Read the model definition and answer for the solid it produces. Units are mm, in the model's axes. Face numbers are marked on the shaded views. Give positions to 0.01 mm unless a question says otherwise; leave off trailing zeros. Order: outer loops, then holes, each group sorted by start corner. A loop starts at its lowest first (then second) coordinate and runs counter-clockwise, first axis right, second up.
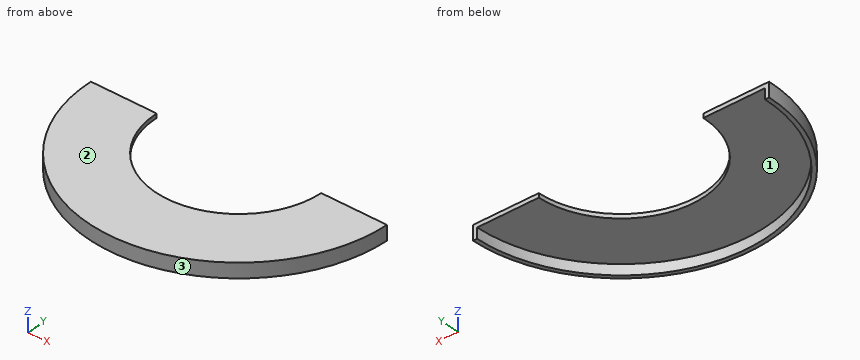
```python
from build123d import *

# Parameters (mm, degrees)
BOSS_EXTRUDE1_DEPTH = 5
BOSS_EXTRUDE2_DEPTH = 2


with BuildPart() as part:
    # Sketch1 → Boss-Extrude1 (new body)
    with BuildSketch(Plane.XY):
        with BuildLine():
            Line((72, 0), (70, 0))
            ThreePointArc((70, 0), (0, -70), (-70, 0))
            Line((-70, 0), (-72, 0))
            ThreePointArc((-72, 0), (0, -72), (72, 0))
        make_face()
    extrude(amount=BOSS_EXTRUDE1_DEPTH)

    # Sketch2 → Boss-Extrude2 (add)
    with BuildSketch(Plane.XY.offset(5)):
        with BuildLine():
            Line((72, 0), (70, 0))
            ThreePointArc((70, 0), (0, -70), (-70, 0))
            Line((-70, 0), (-72, 0))
            ThreePointArc((-72, 0), (0, -72), (72, 0))
        make_face()
        with BuildLine():
            Line((-40, 0), (-70, 0))
            ThreePointArc((-70, 0), (0, -70), (70, 0))
            Line((70, 0), (40, 0))
            ThreePointArc((40, 0), (0, -40), (-40, 0))
        make_face()
    extrude(amount=BOSS_EXTRUDE2_DEPTH)


solid = part.part
```
1) For a pull along X with two mould halves and no side action, classify the marked faces 1, 2 and 3 as released by +X, released by -X, zero draft, split by the parting line, or undercut.
Final values:
face 1: undercut
face 2: zero draft
face 3: split by the parting line
2) The part is cut by section A-A on y = -15.5. Determine the outline of the cut face in (x, z).
Final values:
outline: (-70.31, 0) - (-68.26, 0) - (-68.26, 5) - (-36.87, 5) - (-36.87, 7) - (-70.31, 7) - close; (36.87, 5) - (68.26, 5) - (68.26, 0) - (70.31, 0) - (70.31, 7) - (36.87, 7) - close
3) The part is cut by section C-C on y = -54.5. Determine the outline of the cut face in (x, z), and give its area (3 significant figures).
Final values:
outline: (-47.05, 0) - (-43.93, 0) - (-43.93, 5) - (43.93, 5) - (43.93, 0) - (47.05, 0) - (47.05, 7) - (-47.05, 7) - close
area: 219 mm2
4) The part is cut by section B-B on x = 0. Determine the outline of the cut face in (y, z).
Final values:
outline: (-72, 0) - (-70, 0) - (-70, 5) - (-40, 5) - (-40, 7) - (-72, 7) - close
5) Given pin 1 (21 mm diameter, centred on x = 14, y = -29, fed in from -Z); pin 2 (1.5 mm diameter, centred on x = 32.5, z = 1.5, fed in from +Y); pin 3 (1.5 mm diameter, centred on y = -33, z = 2, fed in from -X), each flat-ended and moving along its own axis, determine where each tip first touches the part or whether it passes through.
Final values:
pin 1: stops at z = 5
pin 2: stops at y = -61.6
pin 3: stops at x = -64.37
6) Consider L1, parallel to Z at x = 59, y = -9; L2, parallel to X at y = -49.5, z = 2; L3, parallel to Y at x = -0.5, z = 5.75. Determine where each line is inside the solid, lowest interval first.
Final values:
L1: z = 5 to 7
L2: x = -52.29 to -49.49, 49.49 to 52.29
L3: y = -72 to -40
7) The part is cut by section D-D on x = -30.5. Determine the outline of the cut face in (y, z).
Final values:
outline: (-65.22, 0) - (-63.01, 0) - (-63.01, 5) - (-25.88, 5) - (-25.88, 7) - (-65.22, 7) - close
